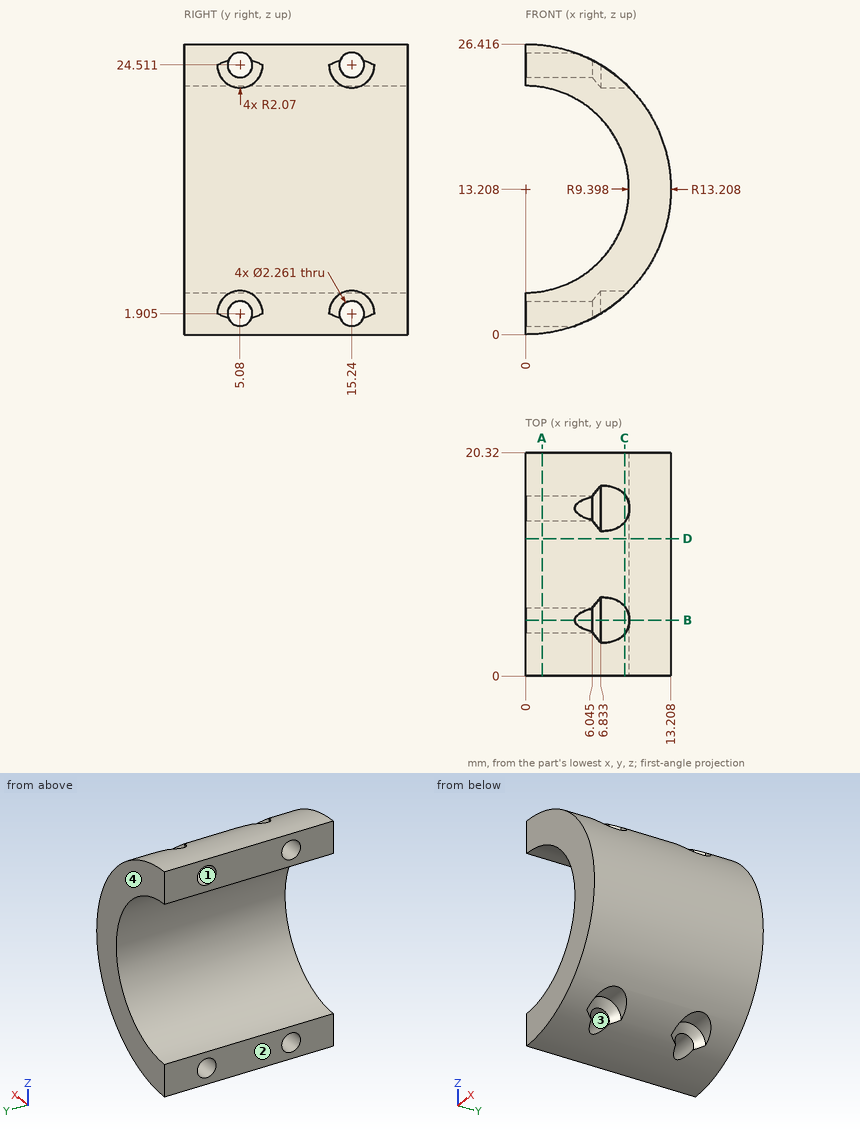
Source: three-view drawing plus pictorial views. Frame: mm from the lowest corner of the part. Coordinates: 2 decimals unless noted, no trailing zeros. Order: outer loops, then holes, each group sorted by start corner. A loop starts at its lowest first (then second) coordinate and runs counter-clockwise, first axis right, second up.
1) Draft query along Y for the marked faces 1, 2, 3 and 4. Return one class per face: released by +Y, released by -Y, zero draft, split by the parting line, or undercut.
Result sheet:
face 1: undercut
face 2: zero draft
face 3: undercut
face 4: released by +Y
2) First-contact query: P1, Ø1.4, axis at y = 5.08, z = 1.905, coming from the -X side; P2, Ø1.5, axis at y = 15, z = 6, coming from the +X side; P3, Ø5, axis at y = 7.5, z = 21.5, coming from the +X side; P4, Ø3, axis at y = 5.08, z = 24.511, coming from the +X side (1 decimal). Flat tips, straight axial feed; report the tip coordinate or a pass-through.
Result sheet:
P1: passes through
P2: stops at x = 11.52
P3: stops at x = 11.87
P4: stops at x = 6.4
3) Ray query, probe 1 along Y at (x, z) = (2.5, 2.25); probe 2 along Z at (x, y) = (3.25, 15.24) (1 decimal); probe 3 along Z at (x, y) = (1, 15.24) (1 decimal). Return the intervals inside material, ascending.
Result sheet:
probe 1: y = 0 to 4, 6.16 to 14.16, 16.32 to 20.32
probe 2: z = 0.4 to 0.8, 3 to 4.4, 22 to 23.4, 25.6 to 26
probe 3: z = 0 to 0.8, 3 to 3.9, 22.6 to 23.4, 25.6 to 26.4
4) Section B-B (y = 5.08). Return loops of the section in (x, z) (1 decimal), then the cut area to 3 significant figures.
Result sheet:
outline: (0, 0) arc R13.2 ccw to (4.5, 0.8) - (0, 0.8) - close; (0, 3) - (6, 3) - (6.8, 4) - (9.4, 4) arc R13.2 ccw to (9.4, 22.4) - (6.8, 22.4) - (6, 23.4) - (0, 23.4) - (0, 22.6) arc R9.4 cw to (0, 3.8) - close; (0, 25.6) - (4.5, 25.6) arc R13.2 ccw to (0, 26.4) - close
area: 100 mm2
5) Section A-A (x = 1.5). Return loops of the section in (y, z) (1 decimal).
Result sheet:
outline: (0, 0.1) - (20.3, 0.1) - (20.3, 3.9) - (0, 3.9) - close; (0, 22.5) - (20.3, 22.5) - (20.3, 26.3) - (0, 26.3) - close; hole circle Ø2.3 at (5.1, 1.9); hole circle Ø2.3 at (5.1, 24.5); hole circle Ø2.3 at (15.2, 1.9); hole circle Ø2.3 at (15.2, 24.5)
6) Section D-D (y = 12.5). Return loops of the section in (x, z), then the cut area to 3 significant figures.
Result sheet:
outline: (0, 0) arc R13.21 ccw to (0, 26.42) - (0, 22.61) arc R9.4 cw to (0, 3.81) - close
area: 135 mm2
7) Section C-C (x = 9). Return loops of the section in (y, z) (1 decimal).
Result sheet:
outline: (0, 3.5) - (3.8, 3.5) arc R2.1 cw to (6.3, 3.5) - (14, 3.5) arc R2.1 cw to (16.5, 3.5) - (20.3, 3.5) - (20.3, 10.5) - (0, 10.5) - close; (0, 15.9) - (20.3, 15.9) - (20.3, 22.9) - (16.5, 22.9) arc R2.1 cw to (14, 22.9) - (6.3, 22.9) arc R2.1 cw to (3.8, 22.9) - (0, 22.9) - close
